from build123d import *

# Parameters (mm, degrees)
CUT_EXTRUDE1_DEPTH = 4
CUT_EXTRUDE2_DEPTH = 3
CHAMFER1_SIZE      = 1
SKETCH4_R          = 3
CUT_EXTRUDE3_DEPTH = 20


with BuildPart() as part:
    # Sketch1 → Revolve1 (revolve)
    with BuildSketch(Plane.XY):
        Polygon((0, 0), (-197, 0), (-197, 12), (-153, 12), (-153, 11), (0, 11), align=None)
    revolve(axis=Axis((0, 0, 0), (-1, 0, 0)))

    # Sketch2 → Cut-Extrude1 (cut)
    with BuildSketch(Plane(origin=(0, 12, 0), x_dir=(1, 0, 0), z_dir=(0, 1, 0))):
        with BuildLine():
            Line((-167.997220054, 4), (-197, 4))
            Line((-197, 4), (-197, -4))
            Line((-197, -4), (-167.997221426, -4))
            ThreePointArc((-167.997221426, -4), (-163.997220054, -6.86e-07), (-167.997220054, 4))
        make_face()
    extrude(amount=-CUT_EXTRUDE1_DEPTH, mode=Mode.SUBTRACT)

    # Sketch3 → Cut-Extrude2 (cut)
    with BuildSketch(Plane(origin=(0, 11, 0), x_dir=(1, 0, 0), z_dir=(0, 1, 0))):
        with BuildLine():
            Line((-147, 3), (0, 3))
            Line((0, 3), (0, -3))
            Line((0, -3), (-147, -3))
            ThreePointArc((-147, -3), (-150, 0), (-147, 3))
        make_face()
    extrude(amount=-CUT_EXTRUDE2_DEPTH, mode=Mode.SUBTRACT)

    # Chamfer1
    chamfer1_edges = [part.edges().sort_by_distance(p)[0] for p in [
        (-197, -12, 0),
        (0, -11, 0),
    ]]
    chamfer(chamfer1_edges, length=CHAMFER1_SIZE)

    # Sketch4 → Cut-Extrude3 (cut)
    with BuildSketch(Plane(origin=(0, 0, 0), x_dir=(0, 0, -1), z_dir=(1, 0, 0))):
        Circle(SKETCH4_R)
    extrude(amount=-CUT_EXTRUDE3_DEPTH, mode=Mode.SUBTRACT)


solid = part.part
Part model, mm, in its own coordinate system. A direction names the side the tool comes from. Give positions to 0.01 mm unless a question says otherwise; leave off trailing zeros. Order: outer loops, then holes, each group sorted by start corner. A loop starts at its lowest first (then second) coordinate and runs counter-clockwise, first axis right, second up. Notation, with made-up numbers: (18.25, 43.25) - (49.25, 43.25) arc R8 cw to (49.25, 57.25) - close; hole circle Ø1 at (72, 62). An arc over 180 degrees is marked (long way). Use a Markdown table: item, result.
1) Saw through at D-D on x = -162. List the corners of the cut face in (y, z), plus the area to 3 significant figures.
Checked values:
| item | result |
|---|---|
| outline | circle Ø24 at (0, 0) |
| area | 452 mm² |
2) 3-axis set-ups, long thin cutter, end or side, ignore diameter. For faces 1 (the cylindrical face through (-164, 10, 0.1)), 2 (the flat face through (0, -3, 2)), 3 (the flat face through (-20, 0, 0)), 4 (the flat face through (-74, 8, 0)), 5 (the cylindrical face through (-174.199, -9.523, 7.302)): which of +Z, -Z, +X, -X, +Y, -Y reach the whole face in a straight line?
Checked values:
| item | result |
|---|---|
| face 1 | -X, +Y |
| face 2 | +Z, -Z, +X, +Y, -Y |
| face 3 | +X |
| face 4 | +X, +Y |
| face 5 | +X, -X |
3) Two-plate mould, pull along Z, no slides. Class faces 6 (the cylindrical face through (-150, 10, 0)), 7 (the flat face through (-153, 5, 10)), 8 (the conical face through (-196.826, -11.165, -0.438)), 9 (the flat face through (-181, 8, 0)): +Z half, -Z half, draft (parallel to the pull), parting line (faces both ways), or undercut.
Checked values:
| item | result |
|---|---|
| face 6 | undercut |
| face 7 | draft |
| face 8 | parting line |
| face 9 | undercut |
4) Probe L1, parallel to Y at x = -4.75, z = 0; L2, parallel to Y at x = -115, z = -0.25; L3, parallel to Z at x = -105.5, y = -9. List the from-to ranges inside material, lowest first. Write a range as from..to.
Checked values:
| item | result |
|---|---|
| L1 | -11..-3, 3..8 |
| L2 | -11..8 |
| L3 | -6.32..6.32 |
5) Saw through at A-A on y = 0. List the corners of the cut face in (x, z).
Checked values:
| item | result |
|---|---|
| outline | (-197, -11) - (-196, -12) - (-153, -12) - (-153, -11) - (-1, -11) - (0, -10) - (0, -3) - (-20, -3) - (-20, 3) - (0, 3) - (0, 10) - (-1, 11) - (-153, 11) - (-153, 12) - (-196, 12) - (-197, 11) - close |
6) Saw through at B-B on z = 0. List the corners of the cut face in (x, y).
Checked values:
| item | result |
|---|---|
| outline | (-197, -11) - (-196, -12) - (-153, -12) - (-153, -11) - (-1, -11) - (0, -10) - (0, -3) - (-20, -3) - (-20, 3) - (0, 3) - (0, 8) - (-150, 8) - (-150, 11) - (-153, 11) - (-153, 12) - (-164, 12) - (-164, 8) - (-197, 8) - close |
7) Saw through at C-C on x = -114. List the corners of the cut face in (y, z), plus the area to 3 significant figures.
Checked values:
| item | result |
|---|---|
| outline | (8, -3) - (8, 3) - (10.58, 3) arc R11 ccw (long way) to (10.58, -3) - close |
| area | 363 mm² |
8) Flat gauge pins, fed straight in: P1, Ø1.7, axis at x = -178.5, y = 9, coming from the +Z side; P2, Ø4, axis at x = -52, z = 6, coming from the -Y side; P3, Ø3, axis at x = -70, y = 1.5, coming from the +Z side; P4, Ø4, axis at y = 8.5, z = 3, coming from the +X side. Where does each tip first touch, or does it go through?
Checked values:
| item | result |
|---|---|
| P1 | z = 8.81 |
| P2 | y = -10.25 |
| P3 | z = 11 |
| P4 | x = 0 |
